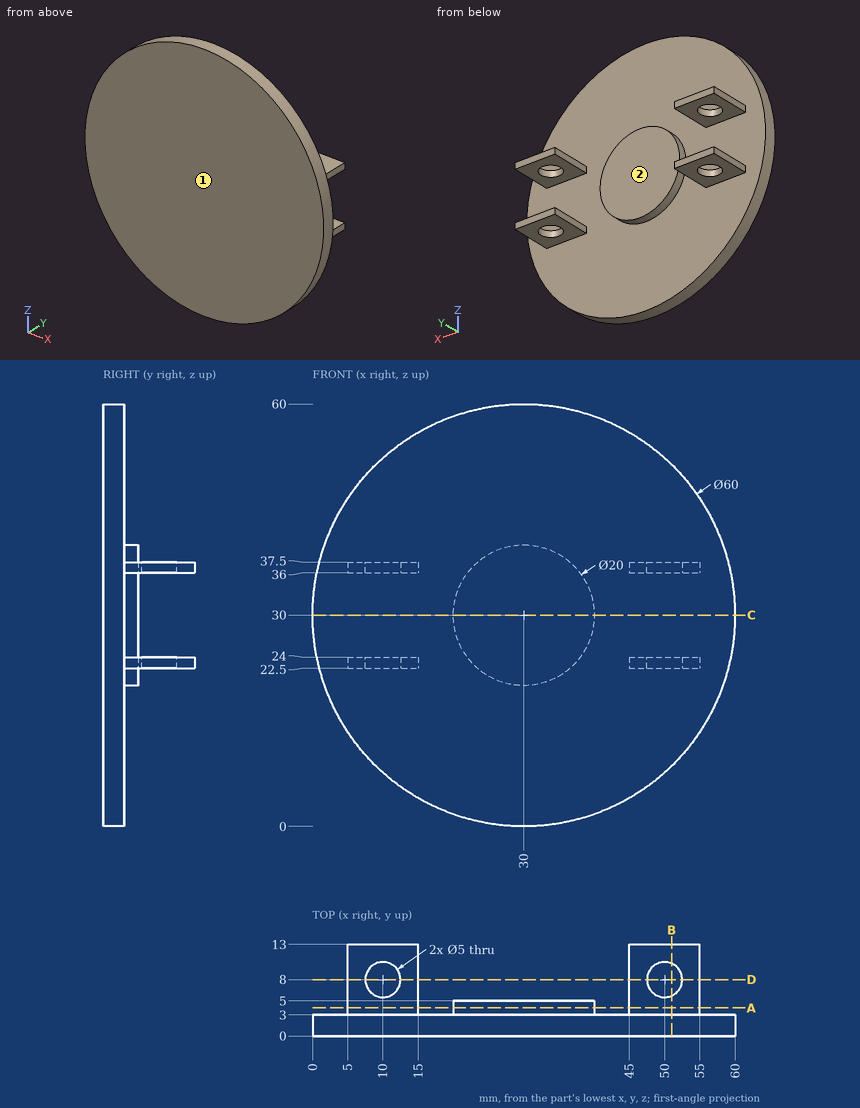
Verification items for this drawing (mm, ordinates from the low corner). A direction names the side the tool comes from. Coordinates: 2 decimals unless noted, no trailing zeros. Order: outer loops, then holes, each group sorted by start corner. A loop starts at its lowest first (then second) coordinate and runs counter-clockwise, first axis right, second up. Notation, with made-up numbers: (21.25, 87) - (56.25, 87) arc R30 ccw to (56.25, 114) - close; hole circle Ø5 at (12.25, -7). An arc over 180 degrees is marked (long way). Answer in a Markdown table with one row per item. Add a question column.
1. Material ranges on L1, parallel to Y at x = 10, z = 37.05; L2, parallel to Z at x = 12.5, y = 9.5; L3, parallel to Y at x = 50, z = 22, recorded low to high. Write a range as [from, to].
2. Section check C-C (z = 30). Enter the section's corners in (x, y).
3. Section check B-B (x = 51). Enter the section's corners in (y, z), plus the area to 3 significant figures.
4. Section check D-D (y = 8). Give the number of separate pieces and of enclosed holes in the cut face, plus the area to 3 significant figures.
5. Gauge pin test, flat ends, axial feed: pin 1 Ø6 at (x, z) = (36, 15) entering from +Y; pin 2 Ø6.5 at (x, y) = (10, 8) entering from -Z; pin 3 Ø6 at (x, y) = (51.5, 10.5) entering from +Z; pin 4 Ø4 at (x, y) = (10, 8) entering from -Z. Record the tip position at first contact, or that the pin passes through.
6. Section check A-A (y = 4). Enter the section's corners in (x, z), plus the area to 3 significant figures.
7. Access from +Z, -Z, +X, -X, +Y, -Y to the whole of each face (thin tool, end or side, straight path). Record for the marked faces 1 and 2.
Data:
| question | item | result |
|---|---|---|
| 1 | L1 | y = [0, 5.5], [10.5, 13] |
| 1 | L2 | z = [22.5, 24], [36, 37.5] |
| 1 | L3 | y = [0, 3] |
| 2 | outline | (0, 0) - (60, 0) - (60, 3) - (40, 3) - (40, 5) - (20, 5) - (20, 3) - (0, 3) - close |
| 3 | outline | (0, 8.58) - (3, 8.58) - (3, 22.5) - (5.71, 22.5) - (5.71, 24) - (3, 24) - (3, 36) - (5.71, 36) - (5.71, 37.5) - (3, 37.5) - (3, 51.42) - (0, 51.42) - close; (10.29, 22.5) - (13, 22.5) - (13, 24) - (10.29, 24) - close; (10.29, 36) - (13, 36) - (13, 37.5) - (10.29, 37.5) - close |
| 3 | area | 145 mm² |
| 4 | separate pieces | 8 |
| 4 | enclosed holes | 0 |
| 4 | area | 30.0 mm² |
| 5 | pin 1 | stops at y = 3 |
| 5 | pin 2 | stops at z = 22.5 |
| 5 | pin 3 | stops at z = 37.5 |
| 5 | pin 4 | passes through |
| 6 | outline | (5, 22.5) - (15, 22.5) - (15, 24) - (5, 24) - close; (5, 36) - (15, 36) - (15, 37.5) - (5, 37.5) - close; circle Ø20 at (30, 30); (45, 22.5) - (55, 22.5) - (55, 24) - (45, 24) - close; (45, 36) - (55, 36) - (55, 37.5) - (45, 37.5) - close |
| 6 | area | 374 mm² |
| 7 | face 1 | +Z, -Z, +X, -X, -Y |
| 7 | face 2 | +Z, -Z, +Y |
